```python
from build123d import *

# Parameters (mm, degrees)
ESTRUSIONE_ESTRUSIONE1_DEPTH           = 5.06
FORO_SVASATO_PER_VITE_M3_2_D           = 3.4
FORO_SVASATO_PER_VITE_M3_2_CSINK_D     = 6.3
FORO_SVASATO_PER_VITE_M3_2_CSINK_ANGLE = 90


with BuildPart() as part:
    # Schizzo4 → Estrusione-Estrusione1 (new body)
    with BuildSketch(Plane.XY):
        with BuildLine():
            Line((-20, 6.4), (0, 0))
            Line((0, 0), (16.02, 0))
            Line((16.02, 0), (29.82, 6.4))
            Line((29.82, 6.4), (29.82, 13.5))
            Line((29.82, 13.5), (25.82, 13.5))
            ThreePointArc((25.82, 13.5), (8.41, 8.1), (-9, 13.5))
            Line((-9, 13.5), (-20, 13.5))
            Line((-20, 13.5), (-20, 6.4))
        make_face()
    extrude(amount=ESTRUSIONE_ESTRUSIONE1_DEPTH)

    # Schizzo7 → Foro filettato M3x0.5-1 (revolve, cut)
    with BuildSketch(Plane(origin=(-20, 10.5, 2.53), x_dir=(0, 0, 1), z_dir=(0, 1, 0))):
        Polygon((0, 0), (0, 9.751075774), (1.25, 9), (1.25, 0), align=None)
    foro_filettato_m3x0_5_1 = revolve(axis=Axis((-26.35, 10.5, 2.53), (1, 0, 0)), mode=Mode.SUBTRACT)

    # Specchia1: Foro filettato M3x0.5-1 across plane
    add(foro_filettato_m3x0_5_1.mirror(Plane.ZY.offset(-4.91)), mode=Mode.SUBTRACT)

    # Foro svasato per Vite M3-2 (through all)
    with Locations(Plane(origin=(-33.438661509, -29.329137282, 5.06), x_dir=(1, 0, 0), z_dir=(0, 0, 1))):
        with Locations((34.605533153, 32.579137282), (48.605533153, 32.579137282)):
            CounterSinkHole(FORO_SVASATO_PER_VITE_M3_2_D / 2, FORO_SVASATO_PER_VITE_M3_2_CSINK_D / 2, counter_sink_angle=FORO_SVASATO_PER_VITE_M3_2_CSINK_ANGLE)


solid = part.part
```
Can you work these out from the model? Positions are in its coordinate system, mm. A direction names the side the tool comes from. Give positions to 0.01 mm unless a question says otherwise; leave off trailing zeros. Order: outer loops, then holes, each group sorted by start corner. A loop starts at its lowest first (then second) coordinate and runs counter-clockwise, first axis right, second up. Notation, with made-up numbers: M 49.5,-2.5 L 64.5,-2.5 A13 ccw 64.5,21.5 Z; hole C 1,14.25 d10. An arc over 180 degrees is marked long. One line per item, written item: value.
1) I want a section at C-C, the plane y = 12.5. List the corners of the cut face in (x, z) for me, plus the area to 3 significant figures.
Answer sheet:
outline: M -20,0 L -7.44,0 L -7.44,5.06 L -20,5.06 Z; M 24.26,0 L 29.82,0 L 29.82,5.06 L 24.26,5.06 Z
area: 91.6 mm^2
2) Please list where these lines run through material, in increasing order: line 1 along Y through (x, z) = (-15.5, 2.53); line 2 along Z through (x, y) = (-17, 10.5); line 3 along Y through (x, z) = (25, 2.53).
Answer sheet:
line 1: y = 4.96 to 9.25, 11.75 to 13.5
line 2: z = 0 to 1.28, 3.78 to 5.06
line 3: y = 4.16 to 9.25, 11.75 to 12.96
3) I want a section at B-B, the plane z = 2.1. Count the separate pieces of the cut face and the enclosed holes in it, plus the area to 3 significant figures.
Answer sheet:
separate pieces: 2
enclosed holes: 2
area: 376 mm^2
4) I want a section at D-D, the plane x = 24.5. List the corners of the cut face in (y, z) for me.
Answer sheet:
outline: M 3.93,0 L 12.64,0 L 12.64,5.06 L 3.93,5.06 Z; hole C 10.5,2.53 d2.5
5) I want a section at A-A, the plane y = 3.25. List the corners of the cut face in (x, z) for me.
Answer sheet:
outline: M -10.16,0 L -0.53,0 L -0.53,3.61 L -1.98,5.06 L -10.16,5.06 Z; M 2.87,0 L 13.47,0 L 13.47,3.61 L 12.02,5.06 L 4.32,5.06 L 2.87,3.61 Z; M 16.87,0 L 23.03,0 L 23.03,5.06 L 18.32,5.06 L 16.87,3.61 Z
6) On a 3-axis mill with a long thin cutter (end or side, diameter ignored), from which of +Z, -Z, +X, -X, +Y, -Y can I reach the whole of each face in a straight line? I mean faces 1 (the face through (29.82, 9, 2)), 2 (the face through (-15.563, 9.446, 3.202)), 3 (the face through (25.38, 9.26, 2.37)). Say none if no direction works.
Answer sheet:
face 1: +Z, -Z, +X, +Y, -Y
face 2: -X
face 3: +X
7) We'd pull the mould along X, two halves only. Please class faces 4 (the face through (-20, 9, 2)), 5 (the face through (13.545, 3.761, 1.78)), 6 (the face through (8, 0, 2)): released by +X, released by -X, zero draft, split by the parting line, or undercut.
Answer sheet:
face 4: released by -X
face 5: undercut
face 6: zero draft
8) For P1, Ø2, axis at y = 10.5, z = 2.53, coming from the +X side, with a flat end and sliding along its axis, tell me the tip position at first contact or that it passes through.
Answer sheet:
P1: stops at x = 20.67
